from build123d import *

# Parameters (mm, degrees)
BOSS_EXTRUDE1_DEPTH = 53
SKETCH2_W           = 9.792899242
SKETCH2_H           = 2.993116411
SKETCH2_H_2         = 2.732466193
BOSS_EXTRUDE2_DEPTH = 2


with BuildPart() as part:
    # Sketch1 → Boss-Extrude1 (new body)
    with BuildSketch(Plane(origin=(0, 0, 0), x_dir=(1, 0, 0), z_dir=(0, 1, 0))):
        with BuildLine():
            Line((-10, 6), (10, 6))
            ThreePointArc((10, 6), (11.414213562, 5.414213562), (12, 4))
            Line((12, 4), (12, -4))
            ThreePointArc((12, -4), (11.414213562, -5.414213562), (10, -6))
            Line((10, -6), (-10, -6))
            ThreePointArc((-10, -6), (-11.414213562, -5.414213562), (-12, -4))
            Line((-12, -4), (-12, 4))
            ThreePointArc((-12, 4), (-11.414213562, 5.414213562), (-10, 6))
        make_face()
    extrude(amount=BOSS_EXTRUDE1_DEPTH)

    # Sketch2 → Boss-Extrude2 (add)
    with BuildSketch(Plane(origin=(0, 53, 0), x_dir=(1, 0, 0), z_dir=(0, 1, 0))):
        with Locations((11.907689601, 3.176051955)):
            Rectangle(SKETCH2_W, SKETCH2_H)
        with Locations((11.907689601, -1.366233097)):
            Rectangle(SKETCH2_W, SKETCH2_H_2)
    extrude(amount=BOSS_EXTRUDE2_DEPTH)


solid = part.part
Input: part model. Units: mm. Frame: model coordinates. A direction names the side the tool comes from. Coordinates: 2 decimals unless noted, no trailing zeros. Loops run counter-clockwise (first coordinate to the right, second up) from the corner with the lowest first, then second, coordinate; pieces in that order, holes last. Notation, with made-up numbers: (76, 85) -> (82, 85) arc R30 ccw to (82, 116) -> close; hole circle Ø3 at (1.5, 55). An arc over 180 degrees is marked (long way). Write each question's results on one line, items separated by ' | '. Start each with the question number.
Q1. Pin query (flat end, axial travel): pin 1 (2 mm diameter, centred on x = 13, y = 54, fed in from -Z); pin 2 (1.6 mm diameter, centred on y = 54.5, z = -3.5, fed in from -X); pin 3 (1.5 mm diameter, centred on x = -1, z = -2.5, fed in from +Y). Return the tip coordinate at first contact, or that it passes through.
Q2. Section C-C, the plane y = 43.5. Return the cut outline in (x, z).
Q3. Section B-B, the plane z = 0.75. Return the cut outline in (x, y).
Q4. Reachability of faces 5 (the cylindrical face through (11.4, 26.13, -5.43)), 6 (the flat face through (7.011, 54, -3)), 7 (the flat face through (12, 54, -4.673)), 8 (the flat face through (14, 53, 1)) from +Z, -Z, +X, -X, +Y, -Y: full face, straight path, thin tool, end or side. Return the list, or none.
Q5. Section A-A, the plane x = 13.25. Return the cut outline in (y, z).
Q6. Ray query, line 1 (X direction, y = 30, z = 0); line 2 (Y direction, x = 4, z = 4.25); line 3 (Z direction, x = -10.5, y = 35). Return the intervals inside material, ascending. Write a range as from..to.
Q7. Pull-direction query (Z, two-part tool) for faces 1 (the flat face through (0, 26, 6)), 2 (the flat face through (0, 26, -6)), 3 (the flat face through (12, 54, 0)), 4 (the flat face through (7.011, 54, 1)); classes: released by +Z, released by -Z, zero draft, split by the parting line, or undercut.
Q8. Section D-D, the plane x = 9. Return the cut outline in (y, z), plus the area to 3 significant figures.
Found:
1) pin 1: z = -4.67 | pin 2: x = 7.01 | pin 3: y = 53
2) outline: (-12, -4) arc R2 ccw to (-10, -6) -> (10, -6) arc R2 ccw to (12, -4) -> (12, 4) arc R2 ccw to (10, 6) -> (-10, 6) arc R2 ccw to (-12, 4) -> close
3) outline: (-12, 0) -> (12, 0) -> (12, 53) -> (16.8, 53) -> (16.8, 55) -> (7.01, 55) -> (7.01, 53) -> (-12, 53) -> close
4) face 5: -Z, +X, -Y | face 6: +Z, -Z, -X, +Y | face 7: -Z, +X, -X, +Y | face 8: +Z, -Z, +X, -Y
5) outline: (53, -4.67) -> (55, -4.67) -> (55, -1.68) -> (53, -1.68) -> close; (53, 0) -> (55, 0) -> (55, 2.73) -> (53, 2.73) -> close
6) line 1: -12..12 | line 2: 0..53 | line 3: -5.94..5.94
7) face 1: released by +Z | face 2: released by -Z | face 3: undercut | face 4: zero draft
8) outline: (0, -6) -> (53, -6) -> (53, -4.67) -> (55, -4.67) -> (55, -1.68) -> (53, -1.68) -> (53, 0) -> (55, 0) -> (55, 2.73) -> (53, 2.73) -> (53, 6) -> (0, 6) -> close | area: 647 mm2
